The listing builds one solid part. Answer for the finished solid, in the listing's coordinates (mm). A direction names the side the tool comes from. Coordinates: 2 decimals unless noted, no trailing zeros. Loops run counter-clockwise (first coordinate to the right, second up) from the corner with the lowest first, then second, coordinate; pieces in that order, holes last. Notation, with made-up numbers: M -12,9.5 L 14,9.5 A28 ccw 14,47.5 Z; hole C 70.5,78 d5. An arc over 180 degrees is marked long. Answer in a Markdown table with one row per item. Add a question column.
from build123d import *

# Parameters (mm, degrees)
SKETCH2_R           = 31
BOSS_EXTRUDE1_DEPTH = 20
SKETCH3_R           = 31
SKETCH3_R_2         = 28
BOSS_EXTRUDE2_DEPTH = 5
CUT_EXTRUDE1_START  = -8
SKETCH4_W           = 15
SKETCH4_H           = 15
CUT_EXTRUDE1_DEPTH  = 76
SKETCH5_R           = 2.65
CUT_EXTRUDE2_DEPTH  = 9


with BuildPart() as part:
    # Sketch2 → Boss-Extrude1 (new body)
    with BuildSketch(Plane.XY):
        with BuildLine():
            Line((-60, -47), (-32.953458565, 14.493776892))
            ThreePointArc((-32.953458565, 14.493776892), (0, 36), (32.953458565, 14.493776892))
            Line((32.953458565, 14.493776892), (60, -47))
            Line((60, -47), (-60, -47))
        make_face()
        Circle(SKETCH2_R, mode=Mode.SUBTRACT)
    extrude(amount=BOSS_EXTRUDE1_DEPTH)

    # Sketch3 → Boss-Extrude2 (add)
    with BuildSketch(Plane(origin=(0, 0, 0), x_dir=(-1, 0, 0), z_dir=(0, 0, -1))):
        Circle(SKETCH3_R)
        Circle(SKETCH3_R_2, mode=Mode.SUBTRACT)
    extrude(amount=-BOSS_EXTRUDE2_DEPTH)

    # Sketch4 → Cut-Extrude1 (cut, through all)
    with BuildSketch(Plane.XZ.offset(47).offset(CUT_EXTRUDE1_START)):
        with Locations((-52.5, 10)):
            Rectangle(SKETCH4_W, SKETCH4_H)
        with Locations((52.5, 10)):
            Rectangle(SKETCH4_W, SKETCH4_H)
    extrude(amount=-CUT_EXTRUDE1_DEPTH, mode=Mode.SUBTRACT)

    # Sketch5 → Cut-Extrude2 (cut, through all)
    with BuildSketch(Plane(origin=(0, -39, 0), x_dir=(1, 0, 0), z_dir=(0, 1, 0))):
        with Locations((-50.740697332, -10)):
            Circle(SKETCH5_R)
        with Locations((50.740697332, -10)):
            Circle(SKETCH5_R)
    extrude(amount=-CUT_EXTRUDE2_DEPTH, mode=Mode.SUBTRACT)


solid = part.part
(1) A cutting plane is placed at A-A (z = 10). Give the vertices of the cut face in (x, y), plus the area to 3 significant figures.
(2) A cutting plane is placed at C-C (y = 0). Give the vertices of the cut face in (x, z).
(3) For faces 5 (the face through (-48, -32, 17.5)), 6 (the face through (1, -47, 10)), 7 (the face through (-48.29, -42.94, 11.01)), 8 (the face through (45, -26, 10)), 9 (the face through (7, -27.4, 5)), determine the directions among +Z, -Z, +X, -X, +Y, -Y from which every point of the face is accessible in a straight line to the end or side of a thin tool.
(4) A cutting plane is placed at B-B (x = 0). Give the vertices of the cut face in (y, z), plus the area to 3 significant figures.
(5) The mould has two halves that part along Y. Classify faces 1 (the face through (-43.66, -9.85, 9.86)), 2 (the face through (-4.036, 30.736, 12.395)), 3 (the face through (-25.865, -10.724, 2.465)), 4 (the face through (1, -33, 0)): released by +Y, released by -Y, zero draft, split by the parting line, or undercut.
(6) A cutting plane is placed at D-D (y = -33). Give the vertices of the cut face in (x, z), plus the area to 3 significant figures.
(7) Straight lines are drawn through the part: line 1 (X direction, y = -44.75, z = 10); line 2 (X direction, y = -42.25, z = 10); line 3 (X direction, y = 28, z = 7). For each, find the intervals that lie inside material, in ascending order.
(8) Each of these flat-tipped pins is pushed along its axis until it touches: pin 1 (1 mm diameter, centred on y = 22.5, z = 8.5, fed in from -X); pin 2 (3.5 mm diameter, centred on x = -52.5, z = 7.5, fed in from +Y); pin 3 (1 mm diameter, centred on x = 1, z = 6.5, fed in from +Y). Where does it stop, or does it pass through?
Solved:
| question | item | result |
|---|---|---|
| 1 | outline | M -60,-47 L -53.39,-47 L -53.39,-39 L -56.48,-39 Z; M -48.09,-47 L 48.09,-47 L 48.09,-39 L 45,-39 L 45,-12.9 L 32.95,14.49 A36 ccw -32.95,14.49 L -45,-12.9 L -45,-39 L -48.09,-39 Z; M 53.39,-47 L 60,-47 L 56.48,-39 L 53.39,-39 Z; hole C 0,0 d62 |
| 1 | area | 3,330 mm² |
| 2 | outline | M -39.33,0 L -28,0 L -28,5 L -31,5 L -31,20 L -39.33,20 Z; M 28,0 L 39.33,0 L 39.33,20 L 31,20 L 31,5 L 28,5 Z |
| 3 | face 5 | -X, +Y |
| 3 | face 6 | +Z, -Z, +X, -X, -Y |
| 3 | face 7 | +Y, -Y |
| 3 | face 8 | +X, +Y |
| 3 | face 9 | +Z |
| 4 | outline | M -47,0 L -28,0 L -28,5 L -31,5 L -31,20 L -47,20 Z; M 28,0 L 36,0 L 36,20 L 31,20 L 31,5 L 28,5 Z |
| 4 | area | 450 mm² |
| 5 | face 1 | released by +Y |
| 5 | face 2 | undercut |
| 5 | face 3 | undercut |
| 5 | face 4 | zero draft |
| 6 | outline | M -53.84,0 L 53.84,0 L 53.84,2.5 L 45,2.5 L 45,17.5 L 53.84,17.5 L 53.84,20 L -53.84,20 L -53.84,17.5 L -45,17.5 L -45,2.5 L -53.84,2.5 Z |
| 6 | area | 1,890 mm² |
| 7 | line 1 | x = -59.01 to -53.39, -48.09 to 48.09, 53.39 to 59.01 |
| 7 | line 2 | x = -57.91 to -53.39, -48.09 to 48.09, 53.39 to 57.91 |
| 7 | line 3 | x = -22.63 to -13.3, 13.3 to 22.63 |
| 8 | pin 1 | stops at x = -28.5 |
| 8 | pin 2 | stops at y = -39 |
| 8 | pin 3 | stops at y = 36 |
